Here's how the part is built. I have some questions about the finished solid (model axes, mm). Face numbers are marked on the shaded views. Round coordinates to 2 decimals unless told otherwise and drop trailing zeros. Loops run counter-clockwise (first coordinate to the right, second up) from the corner with the lowest first, then second, coordinate; pieces in that order, holes last. Notation, with made-up numbers: M -27.5,82 L 19.5,82 A31 cw 19.5,110 Z; hole C 74,-17.5 d7. An arc over 180 degrees is marked long. Use a Markdown table: item, result.
Autodesk Fusion 360 part; units mm, degrees
sketch "Sketch1" plane through (0, 0, 0) normal (0, 0, 1) x (1, 0, 0)
  circle A0 centre (0, 0) radius 13
  circle A1 centre (0, 0) radius 22.5
  circle A2 centre (0, 0) radius 38
  dimension "d1" = 45
  dimension "d2" = 26
  dimension "d3" = 76
extrude "Extrude1" add sketch "Sketch1" along normal blind 20 contours A1
sketch "Sketch2" plane through (0, 0, 0) normal (0, 0, 1) x (1, 0, 0)
  circle A0 centre (0.2654, -30.1553) radius 2.5
  dimension "d8" = 5
extrude "Extrude4" add sketch "Sketch1" along normal blind 20 contours A1 | A2
extrude "Extrude5" cut sketch "Sketch2" along normal blind 6.312
pattern_circular "C-Pattern2" count 3 over 360 about axis through (0, 0, 20) along (0, 0, 1) of "Extrude5"
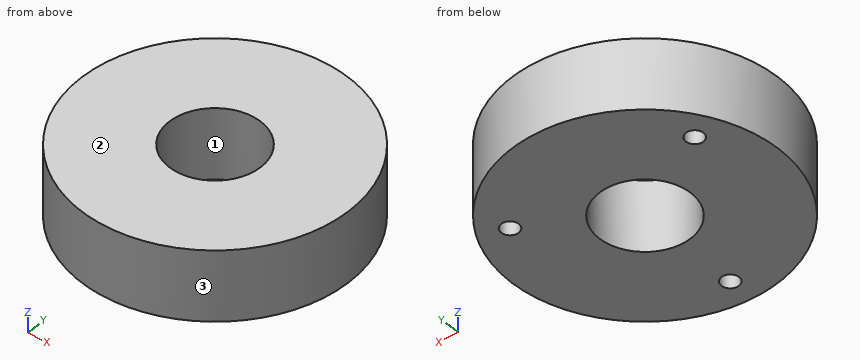
1. Imagine slicing it at B-B, the plane x = 0. Write out the boundary of the cut face in (y, z), then the cut area to 3 significant figures.
Answer sheet:
| item | result |
|---|---|
| outline | M -38,0 L -32.64,0 L -32.64,6.31 L -27.67,6.31 L -27.67,0 L -13,0 L -13,20 L -38,20 Z; M 13,0 L 38,0 L 38,20 L 13,20 Z |
| area | 969 mm2 |
2. Imagine slicing it at D-D, the plane y = -31.5. Write out the boundary of the cut face in (x, z).
Answer sheet:
| item | result |
|---|---|
| outline | M -21.25,0 L -1.84,0 L -1.84,6.31 L 2.37,6.31 L 2.37,0 L 21.25,0 L 21.25,20 L -21.25,20 Z |
3. We'd pull the mould along X, two halves only. Please class the marked faces 1, 2 and 3: +X half, -X half, draft (parallel to the pull), parting line (faces both ways), or undercut.
Answer sheet:
| item | result |
|---|---|
| face 1 | undercut |
| face 2 | draft |
| face 3 | parting line |
4. I need wall thicknesses on probe 1 along Y at (x, z) = (0.5, 15.5); probe 2 along X at (y, z) = (4.5, 3.25); probe 3 along Y at (x, z) = (-7, 4.75). Which ranges of each line are inside material? Lowest first, please. Write a range as from..to.
Answer sheet:
| item | result |
|---|---|
| probe 1 | -38..-12.99, 12.99..38 |
| probe 2 | -37.73..-12.2, 12.2..37.73 |
| probe 3 | -37.35..-10.95, 10.95..37.35 |
5. Imagine slicing it at C-C, the plane z = 9. Write out the boundary of the cut face in (x, y), then the cut area to 3 significant figures.
Answer sheet:
| item | result |
|---|---|
| outline | C 0,0 d76; hole C 0,0 d26 |
| area | 4,010 mm2 |
6. Imagine slicing it at A-A, the plane y = 0. Write out the boundary of the cut face in (x, z), then the cut area to 3 significant figures.
Answer sheet:
| item | result |
|---|---|
| outline | M -38,0 L -13,0 L -13,20 L -38,20 Z; M 13,0 L 38,0 L 38,20 L 13,20 Z |
| area | 1,000 mm2 |
7. For pin 1 Ø2 at (x, z) = (5, 14) entering from -Y; pin 2 Ø23.5 at (x, y) = (0, 0) entering from +Z; pin 3 Ø10 at (y, z) = (-22.5, 2) entering from -X; pin 4 Ø3 at (y, z) = (2.5, 11.5) entering from +X, each with a flat end and sliding along its axis, tell me the tip position at first contact or that it passes through.
Answer sheet:
| item | result |
|---|---|
| pin 1 | y = -37.79 |
| pin 2 | through |
| pin 3 | x = -33.73 |
| pin 4 | x = 37.99 |
